Source: CAD feature listing. Evaluate the final solid. Frame: model axes, mm. Give positions to 0.01 mm unless a question says otherwise; leave off trailing zeros. Write each loop counter-clockwise with the first axis right and the second up, starting at its lowest first coordinate (ties: lowest second). Pieces come first, ordered by that corner, then holes.
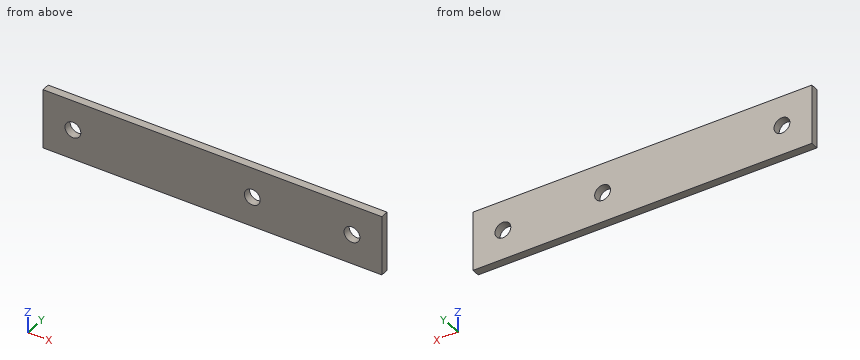
```python
from build123d import *

# Parameters (mm, degrees)
SKETCH1_W           = 68
SKETCH1_H           = 12
SKETCH1_R           = 1.5875
BOSS_EXTRUDE1_DEPTH = 0.79375


with BuildPart() as part:
    # Sketch1 → Boss-Extrude1 (new, symmetric)
    with BuildSketch(Plane(origin=(0, 0, 0), x_dir=(1, 0, 0), z_dir=(0, 1, 0))):
        Rectangle(SKETCH1_W, SKETCH1_H)
        with Locations(Location((-28, 0, 0), (0, 0, 270))):
            Circle(SKETCH1_R, mode=Mode.SUBTRACT)
        with Locations(Location((28, 0, 0), (0, 0, 270))):
            Circle(SKETCH1_R, mode=Mode.SUBTRACT)
        with Locations(Location((8, 0, 0), (0, 0, 270))):
            Circle(SKETCH1_R, mode=Mode.SUBTRACT)
    extrude(amount=BOSS_EXTRUDE1_DEPTH, both=True)


solid = part.part
```
1. Cut plane B-B, the plane z = 0. Return the cut outline in (x, y).
2. Cut plane C-C, the plane y = -0.35. Return the cut outline in (x, z) (1 decimal), then the cut area to 3 significant figures.
3. Cut plane A-A, the plane x = 8. Return the cut outline in (y, z).
4. Line query: L1, parallel to X at y = -0.25, z = 0; L2, parallel to X at y = 0.35, z = -0.5. Output: solid intervals per line, ascending.
Response values:
1. outline: (-34, -0.79) - (-29.59, -0.79) - (-29.59, 0.79) - (-34, 0.79) - close; (-26.41, -0.79) - (6.41, -0.79) - (6.41, 0.79) - (-26.41, 0.79) - close; (9.59, -0.79) - (26.41, -0.79) - (26.41, 0.79) - (9.59, 0.79) - close; (29.59, -0.79) - (34, -0.79) - (34, 0.79) - (29.59, 0.79) - close
2. outline: (-34, -6) - (34, -6) - (34, 6) - (-34, 6) - close; hole circle Ø3.2 at (-28, 0); hole circle Ø3.2 at (8, 0); hole circle Ø3.2 at (28, 0)
2. area: 792 mm2
3. outline: (-0.79, -6) - (0.79, -6) - (0.79, -1.59) - (-0.79, -1.59) - close; (-0.79, 1.59) - (0.79, 1.59) - (0.79, 6) - (-0.79, 6) - close
4. L1: x = -34 to -29.59, -26.41 to 6.41, 9.59 to 26.41, 29.59 to 34
4. L2: x = -34 to -29.51, -26.49 to 6.49, 9.51 to 26.49, 29.51 to 34
